Input: part model. Units: mm. Frame: model coordinates. A direction names the side the tool comes from. Round coordinates to 2 decimals unless told otherwise and drop trailing zeros. Loops run counter-clockwise (first coordinate to the right, second up) from the corner with the lowest first, then second, coordinate; pieces in that order, holes last. Notation, with made-up numbers: M -1,-5.5 L 34,-5.5 A25 ccw 34,29.5 Z; hole C -8.75,72 d9. An arc over 180 degrees is marked long. Return JSON: item names as keys, results as strings. Group by question number.
1) Contact query for flat-ended pins moving along their axis: P1, Ø2, axis at x = 11, z = -2, coming from the +Y side; P2, Ø4.5, axis at y = 2.5, z = 1.5, coming from the -X side; P3, Ø4, axis at y = 18, z = 2.5, coming from the -X side. Output: stop coordinate, or through.
2) Section C-C (x = -11). Output: boundary loops of the cut face in (y, z), plus the area to 3 significant figures.
3) Mould query, pull axis Y, two halves, no side actions, for faces 5 (the face through (0, 0, 0)), 6 (the face through (12, 4, 0)), 7 (the face through (-16.553, 29.501, -0.056)). Classes: +Y half, -Y half, draft (parallel to the pull), parting line (faces both ways), or undercut.
4) Material intervals for line 1 (Y direction, x = -12, z = 0.75) (3 decimals); line 2 (Y direction, x = -11, z = -2.25); line 3 (X direction, y = 28, z = -1), sorted ascending. Write a range as from..to.
5) Section A-A (y = 27). Output: boundary loops of the cut face in (x, z).
6) Section D-D (y = 3.5). Output: boundary loops of the cut face in (x, z).
7) Section B-B (z = 1.75). Output: boundary loops of the cut face in (x, y).
8) Access query for faces 1 (the face through (-10.448, 26.264, -0.07)), 2 (the face through (14.54, 24.86, -0.07)), 3 (the face through (14, 2, 0)), 4 (the face through (-14.313, 24.716, -0.07)). Directions: +Z, -Z, +X, -X, +Y, -Y. A direction counts if a zero-diameter tool reaches every point of the face in a straight line with its end or side. Return the directions, or none.
from build123d import *

# Parameters (mm, degrees)
SKETCH1_W           = 28
SKETCH1_H           = 10
BOSS_EXTRUDE1_DEPTH = 4
BOSS_EXTRUDE2_START = -5
BOSS_EXTRUDE2_DEPTH = 10
FILLET3_R           = 1


with BuildPart() as part:
    # Sketch1 → Boss-Extrude1 (new body)
    with BuildSketch(Plane(origin=(0, 0, 0), x_dir=(1, 0, 0), z_dir=(0, 1, 0))):
        Rectangle(SKETCH1_W, SKETCH1_H)
    extrude(amount=BOSS_EXTRUDE1_DEPTH)

    # Sketch3 → Boss-Extrude2 (add)
    with BuildSketch(Plane.XY.offset(BOSS_EXTRUDE2_START)):
        with BuildLine():
            Line((6.804916492, 22.043099096), (15.434965947, 30.824064473))
            Line((15.434965947, 30.824064473), (17.72994071, 28.10787731))
            Line((17.72994071, 28.10787731), (11.921630408, 22.197995574))
            ThreePointArc((11.921630408, 22.197995574), (0.285107603, 0.121770207), (-11.627623737, 22.050181492))
            Line((-11.627623737, 22.050181492), (-17.72994071, 28.10787731))
            Line((-17.72994071, 28.10787731), (-15.255675803, 31.036260962))
            Line((-15.255675803, 31.036260962), (-6.295168075, 22.141273955))
            ThreePointArc((-6.295168075, 22.141273955), (0.119840794, 4.073834753), (6.804916492, 22.043099096))
        make_face()
    extrude(amount=BOSS_EXTRUDE2_DEPTH)

    # Fillet3
    fillet3_edges = [part.edges().sort_by_distance(p)[0] for p in [
        (16.582453328, 29.465970891, -5),
        (17.72994071, 28.10787731, 0),
        (15.434965947, 30.824064473, 0),
        (-16.492808256, 29.572069136, -5),
        (-15.255675803, 31.036260962, 0),
        (-17.72994071, 28.10787731, 0),
        (16.582453328, 29.465970891, 5),
        (-16.492808256, 29.572069136, 5),
    ]]
    fillet(fillet3_edges, radius=FILLET3_R)


solid = part.part
Returned:
{
 "1": {"P1": "stops at y = 27.33", "P2": "stops at x = -14", "P3": "stops at x = -13.85"},
 "2": {"outline": "M 0,-5 L 4,-5 L 4,5 L 0,5 Z; M 5.62,-5 L 26.81,-5 L 26.81,5 L 5.62,5 Z", "area": "252 mm^2"},
 "3": {"face 5": "-Y half", "face 6": "undercut", "face 7": "+Y half"},
 "4": {"line 1": "y = 0..4, 7.095..21.452, 22.42..27.804", "line 2": "y = 0..4, 5.62..26.81", "line 3": "x = -17.36..-12.2, 12.66..17.37"},
 "5": {"outline": "M -16.61,-5 L -11.19,-5 L -11.19,5 L -16.61,5 Z; M 11.68,-5 L 16.64,-5 L 16.64,5 L 11.68,5 Z"},
 "6": {"outline": "M -14,-5 L 14,-5 L 14,5 L -14,5 Z"},
 "7": {"outline": "M -17.13,28.81 A1 ccw -17.07,27.46 L -11.63,22.05 A14.15 ccw -9.54,4 L -14,4 L -14,0 L 14,0 L 14,4 L 9.93,4 A14.15 ccw 11.92,22.2 L 17.09,27.46 A1 ccw 17.14,28.8 L 16.14,29.99 A1 ccw 14.67,30.04 L 6.8,22.04 A10.2 cw long -6.3,22.14 L -14.49,30.27 A1 ccw -15.96,30.21 Z"},
 "8": {"face 1": "+Z, -Z, +Y", "face 2": "+Z, -Z, +X", "face 3": "+Z, -Z, +X, -Y", "face 4": "+Z, -Z, -X"}
}
